The model under review builds one solid part; all positions refer to its coordinate system, in mm. Face numbers are marked on the shaded views. A direction names the side the tool comes from. Round coordinates to 2 decimals unless told otherwise and drop trailing zeros. Loops run counter-clockwise (first coordinate to the right, second up) from the corner with the lowest first, then second, coordinate; pieces in that order, holes last. Notation, with made-up numbers: M 29.25,54 L 48.25,54 A16 cw 48.25,83 Z; hole C 0.25,67.25 d3. An arc over 180 degrees is marked long. Use a Markdown table: item, result. Add a question column.
```python
from build123d import *

# Parameters (mm, degrees)
CROQUIS1_W              = 44
CROQUIS1_H              = 44
SALIENTE_EXTRUIR1_DEPTH = 2
CROQUIS2_R              = 12
CROQUIS2_R_2            = 2
CORTAR_EXTRUIR1_DEPTH   = 2
CROQUIS3_W              = 44
CROQUIS3_H              = 38
SALIENTE_EXTRUIR2_DEPTH = 2
CROQUIS4_W              = 44
CROQUIS4_H              = 2
SALIENTE_EXTRUIR3_DEPTH = 29
SALIENTE_EXTRUIR4_DEPTH = 2
SALIENTE_EXTRUIR5_DEPTH = 2
CORTAR_EXTRUIR2_DEPTH   = 44
CROQUIS10_W             = 44
CROQUIS10_H             = 40
SALIENTE_EXTRUIR6_DEPTH = 2
CROQUIS11_R             = 3.25
CORTAR_EXTRUIR3_DEPTH   = 66.055745327


with BuildPart() as part:
    # Croquis1 → Saliente-Extruir1 (new body)
    with BuildSketch(Plane.XY):
        Rectangle(CROQUIS1_W, CROQUIS1_H)
    extrude(amount=SALIENTE_EXTRUIR1_DEPTH)

    # Croquis2 → Cortar-Extruir1 (cut)
    with BuildSketch(Plane.XY.offset(2)):
        Circle(CROQUIS2_R)
        with Locations((-15.5, 15.5)):
            Circle(CROQUIS2_R_2)
        with Locations((15.5, 15.5)):
            Circle(CROQUIS2_R_2)
        with Locations((15.5, -15.5)):
            Circle(CROQUIS2_R_2)
        with Locations((-15.5, -15.5)):
            Circle(CROQUIS2_R_2)
    extrude(amount=-CORTAR_EXTRUIR1_DEPTH, mode=Mode.SUBTRACT)

    # Croquis3 → Saliente-Extruir2 (add)
    with BuildSketch(Plane.XY.offset(2)):
        with Locations((0, -41)):
            Rectangle(CROQUIS3_W, CROQUIS3_H)
    extrude(amount=-SALIENTE_EXTRUIR2_DEPTH)

    # Croquis4 → Saliente-Extruir3 (add)
    with BuildSketch(Plane.XY.offset(2)):
        with Locations((0, -22.5)):
            Rectangle(CROQUIS4_W, CROQUIS4_H)
    extrude(amount=SALIENTE_EXTRUIR3_DEPTH)

    # Croquis5 → Saliente-Extruir4 (add)
    with BuildSketch(Plane.ZY.offset(22)):
        Polygon((2, 22), (42, -60), (2, -60), (0, -60), (0, 22), align=None)
    extrude(amount=SALIENTE_EXTRUIR4_DEPTH)

    # Croquis7 → Saliente-Extruir5 (add)
    with BuildSketch(Plane(origin=(22, 0, 0), x_dir=(0, 0, -1), z_dir=(1, 0, 0))):
        Polygon((0, -60), (-42, -60), (-2, 22), (0, 22), align=None)
    extrude(amount=SALIENTE_EXTRUIR5_DEPTH)

    # Croquis8 → Cortar-Extruir2 (cut)
    with BuildSketch(Plane(origin=(22, 0, 0), x_dir=(0, 0, -1), z_dir=(1, 0, 0))):
        Polygon((-24.195121951, -23.5), (-23.219512195, -21.5), (-31, -21.5), (-31, -23.5), align=None)
    extrude(amount=-CORTAR_EXTRUIR2_DEPTH, mode=Mode.SUBTRACT)

    # Croquis10 → Saliente-Extruir6 (add)
    with BuildSketch(Plane.XZ.offset(60)):
        with Locations((0, 22)):
            Rectangle(CROQUIS10_W, CROQUIS10_H)
    extrude(amount=-SALIENTE_EXTRUIR6_DEPTH)

    # Croquis11 → Cortar-Extruir3 (cut, through all)
    with BuildSketch(Plane(origin=(0, -21.5, 0), x_dir=(1, 0, 0), z_dir=(0, 1, 0))):
        with Locations(Location((-12, -12.609756098, 0), (0, 0, 270))):
            Circle(CROQUIS11_R)
        with Locations(Location((12, -12.609756098, 0), (0, 0, 270))):
            Circle(CROQUIS11_R)
    extrude(amount=-CORTAR_EXTRUIR3_DEPTH, mode=Mode.SUBTRACT)


solid = part.part
```
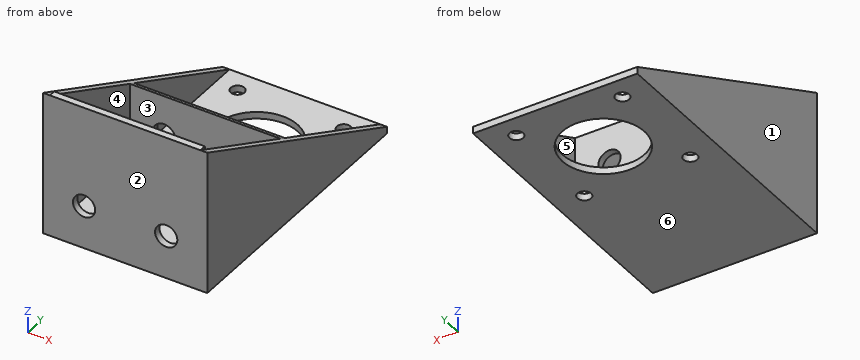
(1) Draft analysis for pull direction Y (two halves, no side actions). For the marked faces 1, 2 and 3, state which applies: released by +Y, released by -Y, zero draft, split by the parting line, or undercut.
(2) Insertion check: pin 1 Ø2.5 at (x, y) = (15.5, -15.5) entering from -Z; pin 2 Ø5 at (x, y) = (15.5, 15.5) entering from +Z; pin 3 Ø7.5 at (x, z) = (12, 12.61) entering from +Y. Each pin has a flat end and moves straight along its axis. Give the tip position at first contact, or say it passes through.
(3) Consider section B-B, the plane z = 12. Give the boundary of the cut face in (x, y).
(4) For the marked faces 4, 5 and 6, list the 3-axis set-ups (+Z, -Z, +X, -X, +Y, -Y) from which the entire face can be reached by the end or side of a thin tool; tool diameter is ignored.
(5) To check wall thickness, follow probe 1 along Y at (x, z) = (-15.5, 0.5); probe 2 along X at (y, z) = (-20, 21.5); probe 3 along Y at (x, z) = (-18.5, 12). State the ranges of each line that lie inside material, in increasing order.
(6) Consider section D-D, the plane z = 28. Give the boundary of the cut face in (x, y), then the cut area to 3 significant figures.
(7) Consider section A-A, the plane x = 0. Give the boundary of the cut face in (y, z), then the cut area to 3 significant figures.
(8) Consider section C-C, the plane y = 0. Give the boundary of the cut face in (x, z).
Found:
| question | item | result |
|---|---|---|
| 1 | face 1 | zero draft |
| 1 | face 2 | released by -Y |
| 1 | face 3 | undercut |
| 2 | pin 1 | passes through |
| 2 | pin 2 | stops at z = 2 |
| 2 | pin 3 | stops at y = -21.5 |
| 3 | outline | M -24,-60 L -15.19,-60 L -15.19,-58 L -22,-58 L -22,-23.5 L -15.19,-23.5 L -15.19,-21.5 L -22,-21.5 L -22,1.5 L -24,1.5 Z; M -8.81,-60 L 8.81,-60 L 8.81,-58 L -8.81,-58 Z; M -8.81,-23.5 L 8.81,-23.5 L 8.81,-21.5 L -8.81,-21.5 Z; M 15.19,-60 L 24,-60 L 24,1.5 L 22,1.5 L 22,-21.5 L 15.19,-21.5 L 15.19,-23.5 L 22,-23.5 L 22,-58 L 15.19,-58 Z |
| 4 | face 4 | +Z |
| 4 | face 5 | +Z, +Y |
| 4 | face 6 | -Z, +X, -X, +Y, -Y |
| 5 | probe 1 | y = -60 to -17.5, -13.5 to 13.5, 17.5 to 22 |
| 5 | probe 2 | x = -24 to -22, 22 to 24 |
| 5 | probe 3 | y = -60 to -58, -23.5 to -21.5 |
| 6 | outline | M -24,-60 L 24,-60 L 24,-31.3 L 22,-31.3 L 22,-58 L -22,-58 L -22,-31.3 L -24,-31.3 Z |
| 6 | area | 203 mm^2 |
| 7 | outline | M -60,0 L -12,0 L -12,2 L -21.5,2 L -21.5,23.22 L -23.5,24.2 L -23.5,2 L -58,2 L -58,42 L -60,42 Z; M 12,0 L 22,0 L 22,2 L 12,2 Z |
| 7 | area | 239 mm^2 |
| 8 | outline | M -24,0 L -12,0 L -12,2 L -22,2 L -22,12.73 L -24,12.73 Z; M 12,0 L 24,0 L 24,12.73 L 22,12.73 L 22,2 L 12,2 Z |
